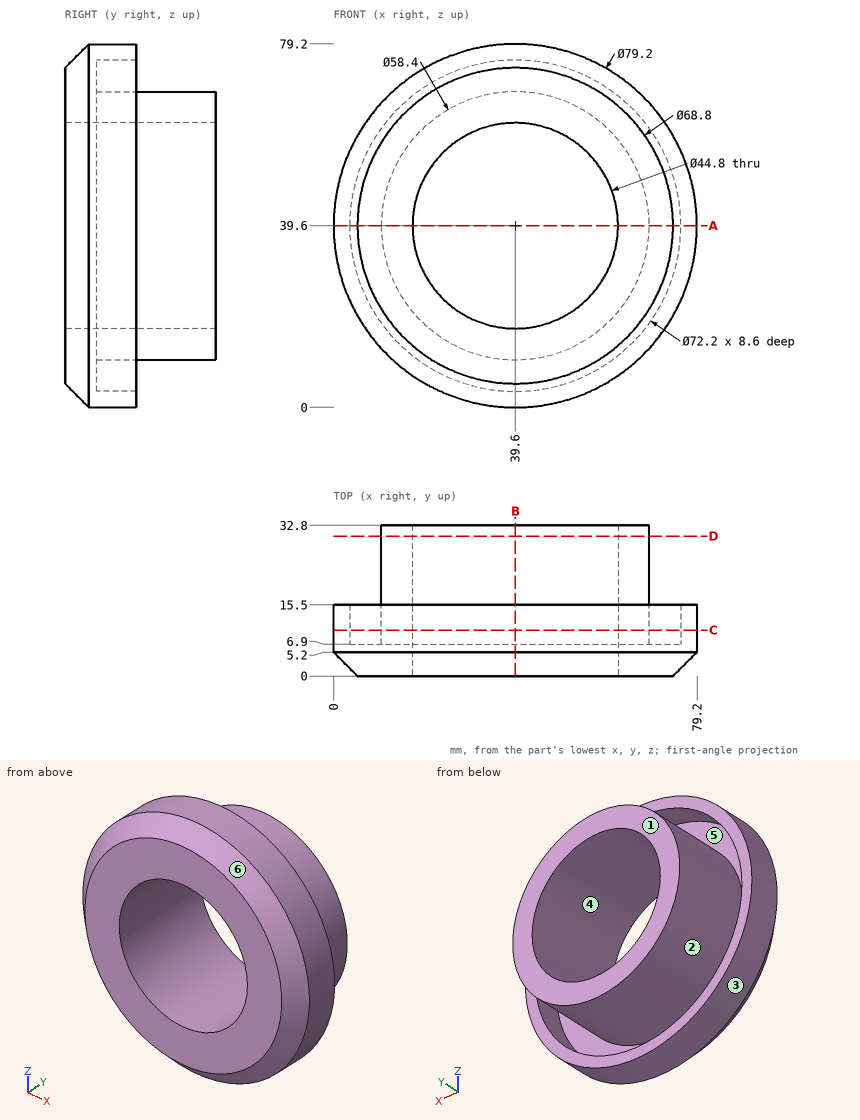
Geometry: see drawing. Coordinates: mm, zero at the bounding-box minimum. A direction names the side the tool comes from. Coordinates: 2 decimals unless noted, no trailing zeros. Loops run counter-clockwise (first coordinate to the right, second up) from the corner with the lowest first, then second, coordinate; pieces in that order, holes last. Notation, with made-up numbers: (9.25, 49.25) -> (27.25, 49.25) arc R13 cw to (27.25, 63.25) -> close; hole circle Ø1 at (-9.75, -16). An arc over 180 degrees is marked (long way). Use a Markdown table: item, result.
1) Cut plane A-A (z = 39.6). Return the cut outline in (x, y).
Results found:
| item | result |
|---|---|
| outline | (0, 5.2) -> (5.2, 0) -> (17.2, 0) -> (17.2, 32.8) -> (10.4, 32.8) -> (10.4, 6.9) -> (3.5, 6.9) -> (3.5, 15.5) -> (0, 15.5) -> close; (62, 0) -> (74, 0) -> (79.2, 5.2) -> (79.2, 15.5) -> (75.7, 15.5) -> (75.7, 6.9) -> (68.8, 6.9) -> (68.8, 32.8) -> (62, 32.8) -> close |
2) Cut plane B-B (x = 39.6). Return the cut outline in (y, z), then the cut area to 3 significant figures.
Results found:
| item | result |
|---|---|
| outline | (0, 5.2) -> (5.2, 0) -> (15.5, 0) -> (15.5, 3.5) -> (6.9, 3.5) -> (6.9, 10.4) -> (32.8, 10.4) -> (32.8, 17.2) -> (0, 17.2) -> close; (0, 62) -> (32.8, 62) -> (32.8, 68.8) -> (6.9, 68.8) -> (6.9, 75.7) -> (15.5, 75.7) -> (15.5, 79.2) -> (5.2, 79.2) -> (0, 74) -> close |
| area | 623 mm2 |
3) Material intervals for line 1 along X through (y, z) = (12, 39); line 2 along Z through (x, y) = (44, 9), sorted ascending. Write a range as from..to.
Results found:
| item | result |
|---|---|
| line 1 | x = 0..3.5, 10.41..17.21, 61.99..68.79, 75.7..79.2 |
| line 2 | z = 0.25..3.77, 10.73..17.64, 61.56..68.47, 75.43..78.95 |
4) Pull-direction query (X, two-part tool) for the marked faces 1, 2, 3 and 4; classes: released by +X, released by -X, zero draft, split by the parting line, or undercut.
Results found:
| item | result |
|---|---|
| face 1 | zero draft |
| face 2 | undercut |
| face 3 | split by the parting line |
| face 4 | undercut |
5) Cut plane C-C (y = 10). Return the cut outline in (x, z).
Results found:
| item | result |
|---|---|
| outline | circle Ø79.2 at (39.6, 39.6); circle Ø58.4 at (39.6, 39.6); hole circle Ø72.2 at (39.6, 39.6); hole circle Ø44.8 at (39.6, 39.6) |
6) Access query for the marked faces 5 and 6. Directions: +Z, -Z, +X, -X, +Y, -Y. A direction counts if a zero-diameter tool reaches every point of the face in a straight line with its end or side. Return the directions, or none.
Results found:
| item | result |
|---|---|
| face 5 | +Y |
| face 6 | -Y |
7) Cut plane D-D (y = 30.5). Return the cut outline in (x, z), then the cut area to 3 significant figures.
Results found:
| item | result |
|---|---|
| outline | circle Ø58.4 at (39.6, 39.6); hole circle Ø44.8 at (39.6, 39.6) |
| area | 1,100 mm2 |
8) Contact query for flat-ended pins moving along their axis: pin 1 (8 mm diameter, centred on x = 45.5, y = 22, fed in from -Z); pin 2 (6 mm diameter, centred on x = 24, z = 47.5, fed in from +Y); pin 3 (10 mm diameter, centred on y = 25, z = 68, fed in from +X); pin 4 (1.5 mm diameter, centred on x = 29.5, y = 13.5, fed in from -Z). Output: stop coordinate, or through.
Results found:
| item | result |
|---|---|
| pin 1 | stops at z = 10.46 |
| pin 2 | passes through |
| pin 3 | stops at x = 57.07 |
| pin 4 | stops at z = 1.12 |
